Here's how the part is built. I have some questions about the finished solid (model axes, mm). A direction names the side the tool comes from. Give positions to 0.01 mm unless a question says otherwise; leave off trailing zeros. Order: outer loops, then holes, each group sorted by start corner. A loop starts at its lowest first (then second) coordinate and runs counter-clockwise, first axis right, second up. Notation, with made-up numbers: (8, 0) -> (18, 0) arc R31 ccw to (18, 35) -> close; hole circle Ø5 at (78.5, -39). An arc over 180 degrees is marked (long way). Write each question's results on one line, items separated by ' | '. Start each with the question number.
Q1. Imagine slicing it at A-A, the plane x = 35. Please give me the cut outline in (y, z).
Q2. Imagine slicing it at D-D, the plane z = -10. Please give me the cut outline in (x, y), then the cut area to 3 significant figures.
Q3. Imagine slicing it at B-B, the plane z = 28. Please give me the cut outline in (x, y), then the cut area to 3 significant figures.
Q4. For faces 1 (the face through (45.9, 27.2, -13.5)), 2 (the face through (48, 3, 11)), 3 (the face through (79, 14, 25.035)), which set-ups out of +Z, -Z, +X, -X, +Y, -Y let a thin tool reach every point of the face, with its end or its side?
Q5. Thinking about a two-plate mould opening in X: for faces 4 (the face through (48, 15, 37)), 5 (the face through (79, 20, 6)), 6 (the face through (15.635, 15, 8)), 7 (the face through (77.784, 14.79, 36.993)), which applies, pulls with the +X half, pulls with the -X half, needs draft (parallel to the pull), parting line crosses it, or undercut?
Q6. I need wall thicknesses on line 1 along Y through (x, z) = (54, 31); line 2 along X through (y, z) = (20.5, 3.5); line 3 along Z through (x, y) = (52.5, 13). Which ranges of each line are inside material? Lowest first, please. Write a range as [from, to].
Q7. Imagine slicing it at C-C, the plane y = 15. Please give me the cut outline in (x, z), then the cut area to 3 significant figures.
Q8. I'm going to push flat-ended pins straight in: pin 1 (1.5 mm diameter, centred on x = 22.5, y = 18, fed in from +Z); pin 2 (12 mm diameter, centred on x = 39.5, y = 12.5, fed in from -Z); pin 3 (1.5 mm diameter, centred on x = 79, y = 12, fed in from -Z). Where does each tip first touch, or does it pass through?
Autodesk Fusion 360 part; units mm, degrees
sketch "Sketch1" plane through (0, 0, 0) normal (0, 1, 0) x (1, 0, 0)
  line L0 (25.6354, -40) -> (70.6354, -40)
  line L1 (80.6354, -30) -> (80.6354, 13.5)
  line L2 (80.6354, 13.5) -> (15.6354, 13.5)
  line L3 (15.6354, 13.5) -> (15.6354, -30)
  arc A0 (15.6354, -30) -> (25.6354, -40) centre (25.6354, -30) ccw
  arc A1 (70.6354, -40) -> (80.6354, -30) centre (70.6354, -30) ccw
  dimension "d1" = 65
  dimension "d2" = 53.5
  dimension "d3" = 10
  dimension "d4" = 10
extrude "Extrude2" add sketch "Sketch1" along normal blind 30
shell "Shell2" thickness 3 removed faces 1 at (58.9688, 20, -13.5)
sketch "Sketch3" plane through (80.6354, 0, 0) normal (1, 0, 0) x (0, 1, 0)
  line L0 (0, 30) -> (0, -13.5)
  line L1 (0, -13.5) -> (30, -13.5)
  line L2 (30, -13.5) -> (30, 30)
  line L3 (30, 30) -> (0, 30)
  line L4 (9, 25.0348) -> (20, 25.0348)
  line L5 (20, 25.0348) -> (20, -16.6958)
  line L6 (20, -16.6958) -> (9, -16.6958)
  line L7 (9, -16.6958) -> (9, 25.0348)
  dimension "d18" = 11
extrude "Extrude4" cut sketch "Sketch3" against normal blind 10 contours L1 L4 L5 L7 | L1 L5 L6 L7
Geometry check:
1) outline: (0, -13.5) -> (3, -13.5) -> (3, 37) -> (27, 37) -> (27, -13.5) -> (30, -13.5) -> (30, 40) -> (0, 40) -> close
2) outline: (15.64, 0) -> (80.64, 0) -> (80.64, 9) -> (77.64, 9) -> (77.64, 3) -> (18.64, 3) -> (18.64, 27) -> (77.64, 27) -> (77.64, 20) -> (80.64, 20) -> (80.64, 30) -> (15.64, 30) -> close | area: 501 mm²
3) outline: (15.64, 0) -> (80.64, 0) -> (80.64, 30) -> (15.64, 30) -> close; hole (18.64, 3) -> (77.64, 3) -> (77.64, 27) -> (18.64, 27) -> close | area: 534 mm²
4) face 1: -Z, +X, -X, +Y, -Y | face 2: -Z | face 3: -Z, +X
5) face 4: undercut | face 5: needs draft | face 6: pulls with the -X half | face 7: pulls with the +X half
6) line 1: [0, 3], [27, 30] | line 2: [15.64, 18.64], [77.64, 80.64] | line 3: [37, 40]
7) outline: (15.64, -13.5) -> (18.64, -13.5) -> (18.64, 30) arc R7 cw to (25.64, 37) -> (70.64, 37) arc R7 cw to (77.64, 30) -> (77.64, 25.03) -> (80.64, 25.03) -> (80.64, 30) arc R10 ccw to (70.64, 40) -> (25.64, 40) arc R10 ccw to (15.64, 30) -> close | area: 361 mm²
8) pin 1: z = 39.71 | pin 2: z = 37 | pin 3: z = 25.03
